```python
from build123d import *

# Parameters (mm, degrees)
IZIM1_W                     = 280
IZIM1_H                     = 100
Y_KSEKLIK_EKSTR_ZYON6_DEPTH = 5
IZIM16_R                    = 8.5
Y_KSEKLIK_EKSTR_ZYON7_DEPTH = 70


with BuildPart() as part:
    # Çizim1 → Yükseklik-Ekstrüzyon6 (new body)
    with BuildSketch(Plane(origin=(0, 0, 0), x_dir=(1, 0, 0), z_dir=(0, 1, 0))):
        with Locations((120, 30)):
            Rectangle(IZIM1_W, IZIM1_H)
    extrude(amount=Y_KSEKLIK_EKSTR_ZYON6_DEPTH)

    # Çizim16 → Yükseklik-Ekstrüzyon7 (add)
    with BuildSketch(Plane(origin=(0, 5, 0), x_dir=(1, 0, 0), z_dir=(0, 1, 0))):
        with Locations(Location((-10, 70, 0), (0, 0, 270))):
            Circle(IZIM16_R)
        with Locations(Location((-10, -10, 0), (0, 0, 90))):
            Circle(IZIM16_R)
        with Locations(Location((250, 69.966428456, 0), (0, 0, 90))):
            Circle(IZIM16_R)
        with Locations(Location((250, -10, 0), (0, 0, 270))):
            Circle(IZIM16_R)
        with Locations(Location((120, 69.966428456, 0), (0, 0, 270))):
            Circle(IZIM16_R)
        with Locations(Location((120, -10, 0), (0, 0, 270))):
            Circle(IZIM16_R)
    extrude(amount=Y_KSEKLIK_EKSTR_ZYON7_DEPTH)


solid = part.part
```
Here's how the part is built. I have some questions about the finished solid (model axes, mm). A direction names the side the tool comes from. Give positions to 0.01 mm unless a question says otherwise; leave off trailing zeros. Write each loop counter-clockwise with the first axis right and the second up, starting at its lowest first coordinate (ties: lowest second). Pieces come first, ordered by that corner, then holes. Notation, with made-up numbers: M -8,87.25 L -4,87.25 A35 ccw -4,125.25 Z; hole C 22,88 d4. An arc over 180 degrees is marked long. Put each result on its own line as item: value. Start each with the question number.
Item 1: If we section it at B-B, the plane z = 10: Write out the boundary of the cut face in (x, y), then the cut area to 3 significant figures.
Item 2: If we section it at C-C, the plane x = 120: Write out the boundary of the cut face in (y, z).
Item 3: Will these pins go through, and if not, where does the flat tip stop? pin 1 (12 mm diameter, centred on y = 35, z = -50, fed in from +X); pin 2 (5 mm diameter, centred on x = 18.5, z = -20.5, fed in from +Y).
Item 4: I need wall thicknesses on L1, parallel to X at y = 49, z = 10.5; L2, parallel to X at y = 49, z = 4; L3, parallel to Y at x = 36, z = -37. Which ranges of each line are inside material? Lowest first, please. Write a range as from..to.
Item 5: Thinking about a two-plate mould opening in X: for faces 3 (the cylindrical face through (-9.63, 39.51, -78.49)), 4 (the flat face through (-10, 75, -70)), 5 (the flat face through (260, 2, -29)), which applies, +X half, -X half, draft (parallel to the pull), parting line (faces both ways), or undercut?
Item 6: If we section it at D-D, the plane z = -69.5: Write out the boundary of the cut face in (x, y), then the cut area to 3 significant figures.
Item 7: On a 3-axis mill with a long thin cutter (end or side, diameter ignored), from which of +Z, -Z, +X, -X, +Y, -Y can I reach the whole of each face in a straight line? I mean faces 1 (the flat face through (250, 75, 10)), 2 (the cylindrical face through (111.7, 39.51, 8.16)). Say none if no direction works.
Item 8: If we section it at A-A, the plane y = 10: Write out the boundary of the cut face in (x, z).
Values:
1. outline: M -20,0 L 260,0 L 260,5 L 258.5,5 L 258.5,75 L 241.5,75 L 241.5,5 L 128.5,5 L 128.5,75 L 111.5,75 L 111.5,5 L -1.5,5 L -1.5,75 L -18.5,75 L -18.5,5 L -20,5 Z
1. area: 4,970 mm²
2. outline: M 0,-80 L 5,-80 L 5,-78.47 L 75,-78.47 L 75,-61.47 L 5,-61.47 L 5,1.5 L 75,1.5 L 75,18.5 L 5,18.5 L 5,20 L 0,20 Z
3. pin 1: through
3. pin 2: y = 5
4. L1: -18.49..-1.51, 111.51..128.49, 241.51..258.49
4. L2: -16.02..-3.98, 113.98..126.02, 243.98..256.02
4. L3: 0..5
5. face 3: undercut
5. face 4: draft
5. face 5: +X half
6. outline: M -20,0 L 260,0 L 260,5 L 258.49,5 L 258.49,75 L 241.51,75 L 241.51,5 L 128.49,5 L 128.49,75 L 111.51,75 L 111.51,5 L -1.51,5 L -1.51,75 L -18.49,75 L -18.49,5 L -20,5 Z
6. area: 4,960 mm²
7. face 1: +Z, -Z, +X, -X, +Y
7. face 2: +Y
8. outline: C -10,-70 d17; C -10,10 d17; C 120,-69.97 d17; C 120,10 d17; C 250,-69.97 d17; C 250,10 d17
